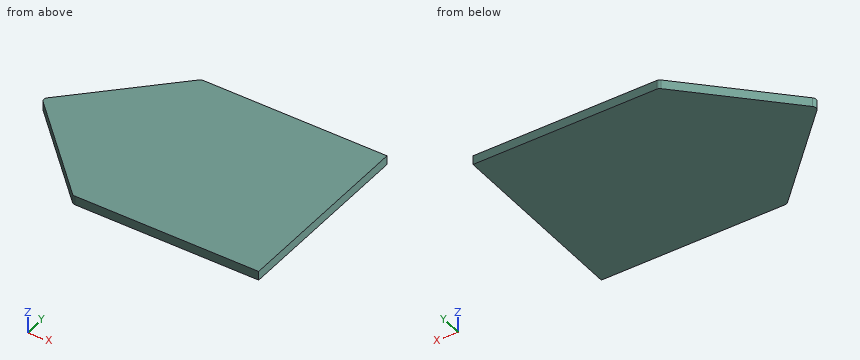
Autodesk Inventor part; units mm, degrees
ref_plane "YZ Plane" through (0, 0, 0) normal (1, 0, 0) x (0, 1, 0)
ref_plane "XZ Plane" through (0, 0, 0) normal (0, 1, 0) x (-1, 0, 0)
ref_plane "XY Plane" through (0, 0, 0) normal (0, 0, 1) x (1, 0, 0)
sketch "Sketch1" plane through (0, 0, 0) normal (0, 0, 1) x (1, 0, 0)
  line L0 (-20.5, 21) -> (20.5, 21)
  line L1 (20.5, 21) -> (20.5, -21)
  line L2 (20.5, -21) -> (-20.5, -21)
  line L3 (-20.5, -21) -> (-20.5, 21) construction
  line L4 (-20.5, 21) -> (20.5, -21) construction
  line L5 (-20.5, -21) -> (-41.5, 0)
  line L6 (-41.5, 0) -> (-20.5, 21)
  point P0 (0, 0)
  point P1 (0, 0)
  point P2 (20.5, 0)
  dimension "d0" = 41
  dimension "d1" = 42
  dimension "d4" = 62
extrude "Plate1" add sketch "Sketch1" along normal blind 2
fillet "Corner Round2" radius 1 3 edges at (-20.5, -21, 1) (-41.5, 0, 1) (-20.5, 21, 1)
equation "\"d2\" = Thickness"
equation "\"BendReliefWidth\" = Thickness"
equation "\"BendReliefDepth\" = 0.5 * Thickness"
equation "\"CornerReliefSize\" = 4 * Thickness"
equation "\"MinimumRemnant\" = 2 * Thickness"
equation "\"TransitionRadius\" = BendRadius"
equation "\"JacobiRadiusSize\" = BendRadius"
equation "\"GapSize\" = Thickness"
properties part number "MNT-CDF-604 CAP" material "Stainless Steel"
Build history of the part. All positions in model axes, mm. Coordinates: 2 decimals unless noted, no trailing zeros. Write each loop counter-clockwise with the first axis right and the second up, starting at its lowest first coordinate (ties: lowest second). Pieces come first, ordered by that corner, then holes.
(1) Cut at A-A on z = 1.55. List the corners of the cut face in (x, y).
(2) Drill centre lines: line 1 (X direction, y = -15.5, z = 0.75); line 2 (X direction, y = -17.5, z = 0.65); line 3 (Y direction, x = -33, z = 0.9). Where is each one in solid material? Low to high.
(3) Pin check, flat tip, straight feed: pin 1 Ø1 at (x, z) = (-24, 1.5) entering from -Y. Stop position of the tip, or through.
(4) Cut at B-B on y = -7.5. List the corners of the cut face in (x, z), and give its area (3 significant figures).
(5) Cut at C-C on x = -34. List the corners of the cut face in (y, z).
Working result:
1. outline: (-40.79, -0.71) - (-20.79, -20.71) arc R1 ccw to (-20.09, -21) - (20.5, -21) - (20.5, 21) - (-20.09, 21) arc R1 ccw to (-20.79, 20.71) - (-40.79, 0.71) arc R1 ccw to start
2. line 1: x = -26 to 20.5
2. line 2: x = -24 to 20.5
2. line 3: y = -8.5 to 8.5
3. pin 1: stops at y = -18
4. outline: (-34, 0) - (20.5, 0) - (20.5, 2) - (-34, 2) - close
4. area: 109 mm2
5. outline: (-7.5, 0) - (7.5, 0) - (7.5, 2) - (-7.5, 2) - close
